Geometry: see drawing. Coordinates: mm, zero at the bounding-box minimum. A direction names the side the tool comes from. Give positions to 0.01 mm unless a question says otherwise; leave off trailing zeros. Loops run counter-clockwise (first coordinate to the right, second up) from the corner with the lowest first, then second, coordinate; pieces in that order, holes last. Notation, with made-up numbers: (21.25, -37.75) - (72.25, -37.75) arc R34 ccw to (72.25, -5.75) - close; hole circle Ø5 at (72, -26.5). An arc over 180 degrees is marked (long way). Use one line per item in the form item = value.
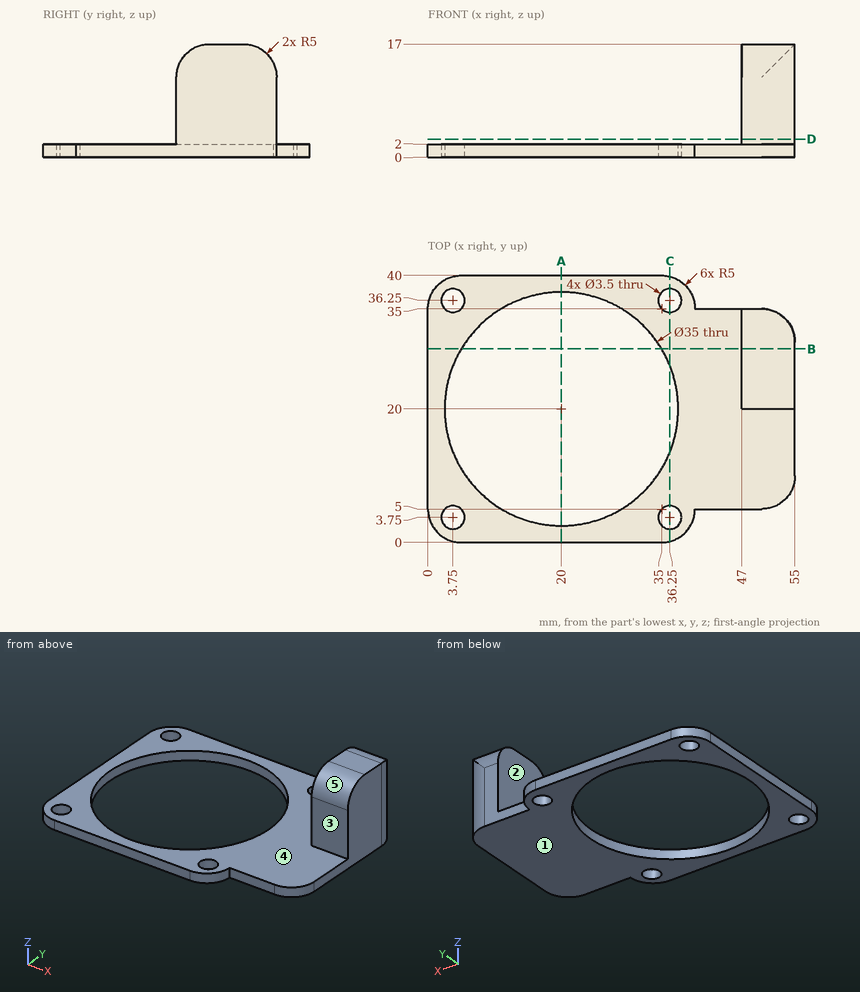
(1) Cut plane A-A (x = 20). Return the cut outline in (y, z), plus the area to 4 significant figures.
Solution:
outline = (0, 0) - (2.5, 0) - (2.5, 2) - (0, 2) - close; (37.5, 0) - (40, 0) - (40, 2) - (37.5, 2) - close
area = 10.00 mm2
(2) Pull-direction query (Y, two-part tool) for the marked faces 4 and 5; classes: released by +Y, released by -Y, zero draft, split by the parting line, or undercut.
Solution:
face_4 = zero draft
face_5 = released by -Y
(3) Material intervals for L1, parallel to Y at x = 20, z = 1; L2, parallel to Z at x = 3, y = 38.5; L3, parallel to X at y = 24.5, z = 14, sorted ascending. Write a range as from..to.
Solution:
L1 = 0..2.5, 37.5..40
L2 = 0..2
L3 = 47..55
(4) Pin query (flat end, axial travel): P1, Ø21, axis at x = 20, y = 20, coming from the +Z side; P2, Ø4, axis at x = 36.25, y = 3.75, coming from the +Z side; P3, Ø2, axis at x = 47.5, z = 1, coming from the -Y side; P4, Ø7.5, axis at y = 25.5, z = 10.5, coming from the -X side. Return the tip coordinate at first contact, or that it passes through.
Solution:
P1 = through
P2 = 2
P3 = 5
P4 = 47
(5) Cut plane B-B (y = 29). Return the cut outline in (x, z), plus the area to 3 significant figures.
Solution:
outline = (0, 0) - (4.99, 0) - (4.99, 2) - (0, 2) - close; (35.01, 0) - (55, 0) - (55, 17) - (47, 17) - (47, 2) - (35.01, 2) - close
area = 170 mm2
(6) Cut plane D-D (z = 2.75). Return the cut outline in (x, y).
Solution:
outline = (47, 20) - (55, 20) - (55, 30) arc R5 ccw to (50, 35) - (47, 35) - close
(7) Cut plane C-C (x = 36.25). Return the cut outline in (y, z), plus the area to 3 significant figures.
Solution:
outline = (0.16, 0) - (2, 0) - (2, 2) - (0.16, 2) - close; (5.5, 0) - (13.5, 0) - (13.5, 2) - (5.5, 2) - close; (26.5, 0) - (34.5, 0) - (34.5, 2) - (26.5, 2) - close; (38, 0) - (39.84, 0) - (39.84, 2) - (38, 2) - close
area = 39.4 mm2
(8) Access query for the marked faces 1, 2 and 3. Directions: +Z, -Z, +X, -X, +Y, -Y. A direction counts if a zero-diameter tool reaches every point of the face in a straight line with its end or side. Return the directions, or none.
Solution:
face_1 = -Z, +X, -X, +Y, -Y
face_2 = +Z, -X, +Y, -Y
face_3 = +Z, +X, -X, -Y
